Design review of the part built by this model. Coordinates are the model's own, in mm. A direction names the side the tool comes from. Coordinates: 2 decimals unless noted, no trailing zeros. Loops run counter-clockwise (first coordinate to the right, second up) from the corner with the lowest first, then second, coordinate; pieces in that order, holes last. Notation, with made-up numbers: M 81,13.25 L 122,13.25 A30 ccw 122,38.25 Z; hole C -30.5,-28 d1. An arc over 180 degrees is marked long. Answer as a JSON object with one key per item and string values. Group by question number.
1. To check wall thickness, follow probe 1 along X at (y, z) = (-7.5, -4); probe 2 along X at (y, z) = (-13.25, 17). State the ranges of each line that lie inside material, in increasing order.
2. Draft analysis for pull direction X (two halves, no side actions). For faces 6 (the flat face through (-0.3, 0.5, 20)), 7 (the cylindrical face through (-19.715, 1.699, -0.266)), 8 (the flat face through (0, -7, 16)), state which applies: +X half, -X half, draft (parallel to the pull), parting line (faces both ways), or undercut.
3. Insertion check: pin 1 (7.5 mm diameter, centred on x = -4.5, y = -8, fed in from -Z); pin 2 (8 mm diameter, centred on x = 5.5, z = -11, fed in from -Y); pin 3 (2 mm diameter, centred on y = -9.5, z = -13.5, fed in from +X). Each pin has a flat end and moves straight along its axis. Give the tip position at first contact, or say it passes through.
4. Consider section D-D (z = 15). State the section outline as (x, y) points.
5. Consider section C-C (y = -5). State the section outline as (x, z) points.
6. Machinability: for faces 1 (the flat face through (-12, 0, 0)), 2 (the flat face through (0, -7, 18)), 3 (the flat face through (0, -7, -18)), 4 (the flat face through (-18, -7, 0)), 5 (the flat face through (11, 1, 0)), which of the approach directions +Z, -Z, +X, -X, +Y, -Y give a long, thin tool a straight path to every point of the face, cutting with its end or side? Answer none if there is none.
7. Consider section B-B (z = -13). State the section outline as (x, y) points, then the cut area to 3 significant figures.
8. Consider section A-A (x = 7.5). State the section outline as (y, z) points, then the cut area to 3 significant figures.
from build123d import *

# Parameters (mm, degrees)
SKETCH1_W           = 40
SKETCH1_H           = 40
SKETCH1_W_2         = 22
SKETCH1_H_2         = 28
BOSS_EXTRUDE1_DEPTH = 2
SKETCH2_W           = 36
SKETCH2_H           = 36
SKETCH2_W_2         = 32
SKETCH2_H_2         = 32
BOSS_EXTRUDE2_DEPTH = 15
FILLET1_R           = 1


with BuildPart() as part:
    # Sketch1 → Boss-Extrude1 (new body)
    with BuildSketch(Plane(origin=(0, 0, 0), x_dir=(1, 0, 0), z_dir=(0, 1, 0))):
        Rectangle(SKETCH1_W, SKETCH1_H)
        Rectangle(SKETCH1_W_2, SKETCH1_H_2, mode=Mode.SUBTRACT)
    extrude(amount=BOSS_EXTRUDE1_DEPTH)

    # Sketch2 → Boss-Extrude2 (add)
    with BuildSketch(Plane(origin=(0, 0, 0), x_dir=(-1, 0, 0), z_dir=(0, -1, 0))):
        Rectangle(SKETCH2_W, SKETCH2_H)
        Rectangle(SKETCH2_W_2, SKETCH2_H_2, mode=Mode.SUBTRACT)
    extrude(amount=BOSS_EXTRUDE2_DEPTH)

    # Fillet1
    fillet1_edges = [part.edges().sort_by_distance(p)[0] for p in [
        (-20, 2, 0),
        (0, 2, 20),
        (20, 2, 0),
        (0, 2, -20),
        (20, 1, 20),
        (-20, 1, 20),
        (-20, 1, -20),
        (20, 1, -20),
    ]]
    fillet(fillet1_edges, radius=FILLET1_R)


solid = part.part
Findings below:
{
 "1": {"probe 1": "x = -18 to -16, 16 to 18", "probe 2": "x = -18 to 18"},
 "2": {"face 6": "draft", "face 7": "-X half", "face 8": "undercut"},
 "3": {"pin 1": "stops at z = -18", "pin 2": "stops at y = 0", "pin 3": "stops at x = 18"},
 "4": {"outline": "M -20,0 L -18,0 L -18,-15 L -16,-15 L -16,0 L 16,0 L 16,-15 L 18,-15 L 18,0 L 20,0 L 20,1 A1 ccw 19,2 L -19,2 A1 ccw -20,1 Z"},
 "5": {"outline": "M -18,-18 L 18,-18 L 18,18 L -18,18 Z; hole M -16,-16 L 16,-16 L 16,16 L -16,16 Z"},
 "6": {"face 1": "-Y", "face 2": "+Z, +X, -X, -Y", "face 3": "-Z, +X, -X, -Y", "face 4": "+Z, -Z, -X, -Y", "face 5": "+Y, -Y"},
 "7": {"outline": "M -20,0 L -18,0 L -18,-15 L -16,-15 L -16,0 L -11,0 L -11,2 L -19,2 A1 ccw -20,1 Z; M 11,0 L 16,0 L 16,-15 L 18,-15 L 18,0 L 20,0 L 20,1 A1 ccw 19,2 L 11,2 Z", "area": "95.6 mm^2"},
 "8": {"outline": "M -15,-18 L 0,-18 L 0,-20 L 1,-20 A1 ccw 2,-19 L 2,-14 L 0,-14 L 0,-16 L -15,-16 Z; M -15,16 L 0,16 L 0,14 L 2,14 L 2,19 A1 ccw 1,20 L 0,20 L 0,18 L -15,18 Z", "area": "83.6 mm^2"}
}
